Source: CAD feature listing. Evaluate the final solid. Frame: model axes, mm. Coordinates: 2 decimals unless noted, no trailing zeros. Order: outer loops, then holes, each group sorted by start corner. A loop starts at its lowest first (then second) coordinate and runs counter-clockwise, first axis right, second up. Notation, with made-up numbers: (14.25, 43) -> (64.25, 43) arc R11 cw to (64.25, 57) -> close; hole circle Ø2 at (34.25, 81). An arc over 180 degrees is marked (long way). Write item = value, one per line. Start each with the question number.
Item 1: Mould query, pull axis Y, two halves, no side actions, for faces 1 (the cylindrical face through (-1.72, -7.75, 12.52)), 2 (the flat face through (2, 2, 25.4)), 3 (the cylindrical face through (-1.926, -0.607, 4.829)). Classes: released by +Y, released by -Y, zero draft, split by the parting line, or undercut.
Item 2: Section query B-B (y = 5.5). Output: boundary loops of the cut face in (x, z).
Item 3: Ray query, line 1 along Y through (x, z) = (0, 4.25); line 2 along Z through (x, y) = (5.5, 0); line 3 along X through (y, z) = (1.25, 8.5). Return the intervals inside material, ascending. Write a range as [from, to].
Item 4: Section query C-C (x = -6.75). Output: boundary loops of the cut face in (y, z).
Item 5: Contact query for flat-ended pins moving along their axis: pin 1 (1 mm diameter, centred on x = -4.5, y = 2, fed in from -Z); pin 2 (1.5 mm diameter, centred on y = 1, z = 17.5, fed in from +X); pin 3 (1 mm diameter, centred on y = -6, z = 15.5, fed in from -X); pin 4 (5 mm diameter, centred on y = 5, z = 6, fed in from +X). Output: stop coordinate, or through.
Item 6: Section query D-D (z = 16). Output: boundary loops of the cut face in (x, y) (1 decimal), then the cut area to 3 significant figures.
Item 7: Section query A-A (z = 8.75). Output: boundary loops of the cut face in (x, y) (1 decimal), then the cut area to 3 significant figures.
```python
from build123d import *

# Parameters (mm, degrees)
F0_R     = 7.9375
F1_DEPTH = 25.4
F4_D     = 4.0386
F4_DEPTH = 9.525
F4_TIP   = 1.213317848
F2_R     = 2.38125
F5_DEPTH = 0.0635


# Not quite as in the source:
# - a length typed as a fraction of an inch, garbled in the dataset ("3 / 203.2 mm" for 3/8 in), is restored


with BuildPart() as f1:
    # F0 (on Top) → F1 (new body)
    with BuildSketch(Plane.XY):
        Circle(F0_R)
    extrude(amount=F1_DEPTH)

    # F4
    with Locations(Plane(origin=(0, 0, 0), x_dir=(1, 0, 0), z_dir=(0, 0, -1))):
        with Locations((0, 0)):
            Hole(F4_D / 2, depth=F4_DEPTH)
            with Locations((0, 0, -(F4_DEPTH + F4_TIP / 2))):  # 118° drill point
                Cone(0, F4_D / 2, F4_TIP, mode=Mode.SUBTRACT)

    # F2 (on face) → F5 (join)
    with BuildSketch(Plane.XY.offset(25.4)):
        Circle(F2_R)
    extrude(amount=F5_DEPTH)


solid = f1.part
```
Computed:
q1.face_1 = split by the parting line
q1.face_2 = zero draft
q1.face_3 = undercut
q2.outline = (-5.72, 0) -> (5.72, 0) -> (5.72, 25.4) -> (-5.72, 25.4) -> close
q3.line_1 = [-7.94, -2.02], [2.02, 7.94]
q3.line_2 = [0, 25.4]
q3.line_3 = [-7.84, -1.59], [1.59, 7.84]
q4.outline = (-4.18, 0) -> (4.18, 0) -> (4.18, 25.4) -> (-4.18, 25.4) -> close
q5.pin_1 = 0
q5.pin_2 = 7.93
q5.pin_3 = -5.72
q5.pin_4 = 7.53
q6.outline = circle Ø15.9 at (0, 0)
q6.area = 198 mm^2
q7.outline = circle Ø15.9 at (0, 0); hole circle Ø4 at (0, 0)
q7.area = 185 mm^2
